```python
from build123d import *

# Parameters (mm, degrees)
SKETCH1_R           = 3.175
EXTRUDE1_DEPTH      = 139.7
CHAMFER1_SIZE       = 0.635
EXTRUDE7_DEPTH      = 140.7
EXTRUDE7_DEPTH_BACK = 140.7


with BuildPart() as part:
    # Sketch1 → Extrude1 (new body, symmetric)
    with BuildSketch(Plane.XY):
        Circle(SKETCH1_R)
    extrude(amount=EXTRUDE1_DEPTH, both=True)

    # Chamfer1
    chamfer1_edges = [part.edges().sort_by_distance(p)[0] for p in [
        (-3.175, 0, -139.7),
        (-3.175, 0, 139.7),
    ]]
    chamfer(chamfer1_edges, length=CHAMFER1_SIZE)

    # Sketch13 → Extrude7 (cut, two sides)
    with BuildSketch(Plane.XY) as extrude7_sk:
        with BuildLine():
            Line((-1.5875, 2.749630657), (1.5875, 2.749630657))
            ThreePointArc((1.5875, 2.749630657), (0, 3.175), (-1.5875, 2.749630657))
        make_face()
    extrude(amount=EXTRUDE7_DEPTH, mode=Mode.SUBTRACT)
    extrude(extrude7_sk.sketch, amount=-EXTRUDE7_DEPTH_BACK, mode=Mode.SUBTRACT)


solid = part.part
```
Check sheet for the modelled part. Datum: model origin and axes. Units: mm. Round coordinates to 2 decimals unless told otherwise and drop trailing zeros. Write item = value, one per line. Start each with the question number.
Q1. Depth check by flat-ended pin: P1, Ø1.5, axis at y = -1, z = -27.5, coming from the -X side; P2, Ø2, axis at y = -1.5, z = -33, coming from the +X side. Enter the tip coordinate at first touch or a pass-through.
Q2. Release check for a two-part mould opening along Y. For faces 1 (the face through (0, 0, 139.7)), 2 (the face through (-0.116, -3.173, 1.947)) record: pulls with the +Y half, pulls with the -Y half, needs draft (parallel to the pull), parting line crosses it, or undercut.
Q3. Thickness scan on L1, parallel to X at y = -0.5, z = 62.5; L2, parallel to X at y = -2.15, z = -9; L3, parallel to Y at x = -1.25, z = 70. Record the ranges inside material, lowest first.
Derived:
q1.P1 = -3.17
q1.P2 = 3.14
q2.face_1 = needs draft
q2.face_2 = parting line crosses it
q3.L1 = -3.14 to 3.14
q3.L2 = -2.34 to 2.34
q3.L3 = -2.92 to 2.75
